Input: part model. Units: mm. Frame: model coordinates. A direction names the side the tool comes from. Round coordinates to 2 decimals unless told otherwise and drop trailing zeros. Write each loop counter-clockwise with the first axis right and the second up, starting at its lowest first coordinate (ties: lowest second). Pieces come first, ordered by that corner, then holes. Notation, with made-up numbers: (17.25, 72) -> (21.25, 72) arc R34 cw to (21.25, 108) -> close; hole circle Ø5 at (-14.75, 73.25). An arc over 180 degrees is marked (long way). Write item = value, one per line.
```python
from build123d import *

# Parameters (mm, degrees)
SKETCH1_W           = 114.3
SKETCH1_H           = 63.5
BOSS_EXTRUDE1_DEPTH = 3.175
SKETCH2_W           = 114.3
SKETCH2_H           = 63.5
SKETCH2_W_2         = 107.95
SKETCH2_H_2         = 57.15
BOSS_EXTRUDE2_DEPTH = 12.7
CUT_EXTRUDE1_REACH  = 69.277
SKETCH3_R           = 3.175
SKETCH3_W           = 63.5
SKETCH3_H           = 4.233333418
SKETCH4_R           = 4.445
SKETCH4_R_2         = 3.175
BOSS_EXTRUDE3_DEPTH = 3.175


with BuildPart() as part:
    # Sketch1 → Boss-Extrude1 (new body)
    with BuildSketch(Plane.XY):
        Rectangle(SKETCH1_W, SKETCH1_H)
    extrude(amount=BOSS_EXTRUDE1_DEPTH)

    # Sketch2 → Boss-Extrude2 (add)
    with BuildSketch(Plane.XY.offset(3.175)):
        Rectangle(SKETCH2_W, SKETCH2_H)
        Rectangle(SKETCH2_W_2, SKETCH2_H_2, mode=Mode.SUBTRACT)
    extrude(amount=BOSS_EXTRUDE2_DEPTH)

    # Sketch3 → Cut-Extrude1 (cut, up to next)
    with BuildSketch(Plane(origin=(0, 0, 0), x_dir=(-1, 0, 0), z_dir=(0, 0, -1)), mode=Mode.PRIVATE) as cut_extrude1_sk1:
        Circle(SKETCH3_R)
    cut_extrude1_tool1 = extrude(cut_extrude1_sk1.sketch, amount=-CUT_EXTRUDE1_REACH, mode=Mode.PRIVATE) & part.part
    # Sketch3 → Cut-Extrude1 (cut, up to next)
    with BuildSketch(Plane(origin=(0, 0, 0), x_dir=(-1, 0, 0), z_dir=(0, 0, -1)), mode=Mode.PRIVATE) as cut_extrude1_sk2:
        with Locations((0, 24.553333291)):
            Rectangle(SKETCH3_W, SKETCH3_H)
    cut_extrude1_tool2 = extrude(cut_extrude1_sk2.sketch, amount=-CUT_EXTRUDE1_REACH, mode=Mode.PRIVATE) & part.part
    # Sketch3 → Cut-Extrude1 (cut, up to next)
    with BuildSketch(Plane(origin=(0, 0, 0), x_dir=(-1, 0, 0), z_dir=(0, 0, -1)), mode=Mode.PRIVATE) as cut_extrude1_sk3:
        with Locations((0, -24.553333291)):
            Rectangle(SKETCH3_W, SKETCH3_H)
    cut_extrude1_tool3 = extrude(cut_extrude1_sk3.sketch, amount=-CUT_EXTRUDE1_REACH, mode=Mode.PRIVATE) & part.part
    add(cut_extrude1_tool1.solids().sort_by_distance((0, 0, 0))[0], mode=Mode.SUBTRACT)
    add(cut_extrude1_tool2.solids().sort_by_distance((0, 24.553333, 0))[0], mode=Mode.SUBTRACT)
    add(cut_extrude1_tool3.solids().sort_by_distance((0, -24.553333, 0))[0], mode=Mode.SUBTRACT)

    # Sketch4 → Boss-Extrude3 (add)
    # profile 1 of 2: a face of its own
    with BuildSketch(Plane.XY.offset(3.175)):
        with Locations(Location((44.45, 0, 0), (0, 0, 180))):
            Circle(SKETCH4_R)
        with Locations((44.45, 0)):
            Circle(SKETCH4_R_2, mode=Mode.SUBTRACT)
    # profile 2 of 2: a face of its own
    with BuildSketch(Plane.XY.offset(3.175)):
        with Locations(Location((-44.45, 0, 0), (0, 0, 180))):
            Circle(SKETCH4_R)
        with Locations(Location((-44.45, 0, 0), (0, 0, 180))):
            Circle(SKETCH4_R_2, mode=Mode.SUBTRACT)
    extrude(amount=BOSS_EXTRUDE3_DEPTH)


solid = part.part
```
1) Line query: L1, parallel to Y at x = -44.45, z = 5.2 (3 decimals); L2, parallel to Y at x = 0, z = 0.7 (3 decimals); L3, parallel to X at y = -12, z = 6 (3 decimals). Output: solid intervals per line, ascending. Write a range as from..to.
Solutions:
L1 = -31.75..-28.575, -4.445..-3.175, 3.175..4.445, 28.575..31.75
L2 = -31.75..-26.67, -22.437..-3.175, 3.175..22.437, 26.67..31.75
L3 = -57.15..-53.975, 53.975..57.15
2) Cut plane A-A (x = 0). Return the cut outline in (y, z) (3 decimals).
Solutions:
outline = (-31.75, 0) -> (-26.67, 0) -> (-26.67, 3.175) -> (-28.575, 3.175) -> (-28.575, 15.875) -> (-31.75, 15.875) -> close; (-22.437, 0) -> (-3.175, 0) -> (-3.175, 3.175) -> (-22.437, 3.175) -> close; (3.175, 0) -> (22.437, 0) -> (22.437, 3.175) -> (3.175, 3.175) -> close; (26.67, 0) -> (31.75, 0) -> (31.75, 15.875) -> (28.575, 15.875) -> (28.575, 3.175) -> (26.67, 3.175) -> close
3) First-contact query: P1, Ø1.9, axis at x = 45.5, y = 0.5, coming from the +Z side (3 decimals); P2, Ø4.5, axis at x = 44, y = 2, coming from the +Z side. Flat tips, straight axial feed; report the tip coordinate or a pass-through.
Solutions:
P1 = 3.175
P2 = 6.35
4) Access query for faces 1 (the face through (-1, 31.75, 8)), 2 (the face through (0, 22.437, 2)), 3 (the face through (53.975, 0, 9)). Directions: +Z, -Z, +X, -X, +Y, -Y. A direction counts if a zero-diameter tool reaches every point of the face in a straight line with its end or side. Return the directions, or none.
Solutions:
face_1 = +Z, -Z, +X, -X, +Y
face_2 = +Z, -Z
face_3 = +Z
5) Cut plane B-B (y = 0). Return the cut outline in (x, z) (3 decimals), and give its area (3 significant figures).
Solutions:
outline = (-57.15, 0) -> (-3.175, 0) -> (-3.175, 3.175) -> (-40.005, 3.175) -> (-40.005, 6.35) -> (-41.275, 6.35) -> (-41.275, 3.175) -> (-47.625, 3.175) -> (-47.625, 6.35) -> (-48.895, 6.35) -> (-48.895, 3.175) -> (-53.975, 3.175) -> (-53.975, 15.875) -> (-57.15, 15.875) -> close; (3.175, 0) -> (57.15, 0) -> (57.15, 15.875) -> (53.975, 15.875) -> (53.975, 3.175) -> (48.895, 3.175) -> (48.895, 6.35) -> (47.625, 6.35) -> (47.625, 3.175) -> (41.275, 3.175) -> (41.275, 6.35) -> (40.005, 6.35) -> (40.005, 3.175) -> (3.175, 3.175) -> close
area = 440 mm^2
6) Cut plane D-D (x = 18.5). Return the cut outline in (y, z) (3 decimals).
Solutions:
outline = (-31.75, 0) -> (-26.67, 0) -> (-26.67, 3.175) -> (-28.575, 3.175) -> (-28.575, 15.875) -> (-31.75, 15.875) -> close; (-22.437, 0) -> (22.437, 0) -> (22.437, 3.175) -> (-22.437, 3.175) -> close; (26.67, 0) -> (31.75, 0) -> (31.75, 15.875) -> (28.575, 15.875) -> (28.575, 3.175) -> (26.67, 3.175) -> close
7) Cut plane C-C (z = 1.25). Return the cut outline in (x, y) (3 decimals), and give its area (3 significant figures).
Solutions:
outline = (-57.15, -31.75) -> (57.15, -31.75) -> (57.15, 31.75) -> (-57.15, 31.75) -> close; hole (-31.75, -26.67) -> (31.75, -26.67) -> (31.75, -22.437) -> (-31.75, -22.437) -> close; hole (-31.75, 22.437) -> (31.75, 22.437) -> (31.75, 26.67) -> (-31.75, 26.67) -> close; hole circle Ø6.35 at (0, 0)
area = 6,690 mm^2
